Part print with two shaded views. Sizes in mm from the minimum x, y, z corner. A direction names the side the tool comes from. Coordinates: 2 decimals unless noted, no trailing zeros. Loops run counter-clockwise (first coordinate to the right, second up) from the corner with the lowest first, then second, coordinate; pieces in that order, holes last. Notation, with made-up numbers: (88.25, 16) -> (125.25, 16) arc R13 cw to (125.25, 40) -> close; hole circle Ø4 at (89, 0.25). An arc over 180 degrees is marked (long way). Write each question's results on one line, items separated by ' | '.
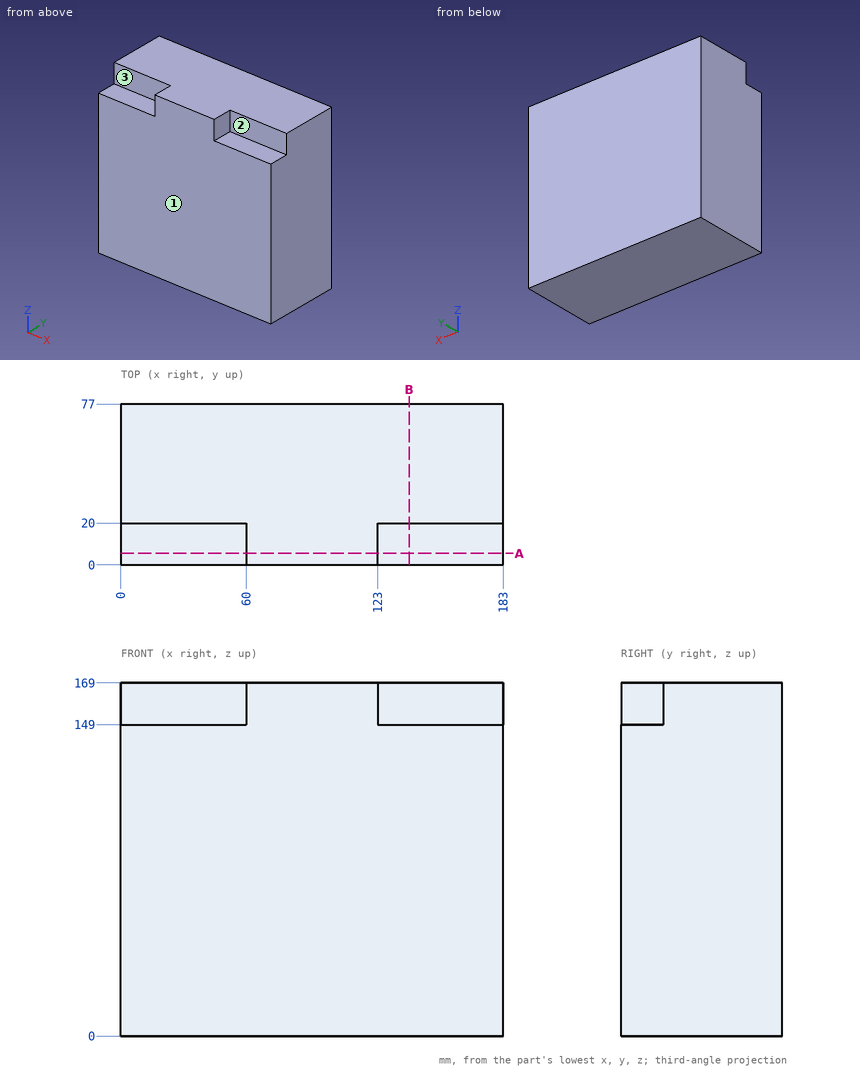
Q1. Which spindle directions (+Z, -Z, +X, -X, +Y, -Y) get a long thin tool onto all of the face, cutting with end or side? Do the marked faces 1, 2 and 3. Say none if no direction does.
Results are:
face 1: +Z, -Z, +X, -X, -Y | face 2: +Z, +X, -Y | face 3: +Z, -X, -Y
Q2. Drop flat-ended pins along their axis: pin 1 (6 mm diameter, centred on y = 12.5, z = 154.5, fed in from -X); pin 2 (22 mm diameter, centred on x = 24, y = 6.5, fed in from +Z); pin 3 (10 mm diameter, centred on y = 13.5, z = 162.5, fed in from +X). Give the stop position or say it passes through.
Results are:
pin 1: x = 60 | pin 2: z = 149 | pin 3: x = 123
Q3. Cut at A-A on y = 5.5. Write the cut outline in (x, z).
Results are:
outline: (0, 0) -> (183, 0) -> (183, 149) -> (123, 149) -> (123, 169) -> (60, 169) -> (60, 149) -> (0, 149) -> close
Q4. Wall check: L1, parallel to Z at x = 176.5, y = 6. Give the ranges that are in metal, low to high. Write a range as from..to.
Results are:
L1: 0..149
Q5. Cut at B-B on x = 138. Write the cut outline in (y, z).
Results are:
outline: (0, 0) -> (77, 0) -> (77, 169) -> (20, 169) -> (20, 149) -> (0, 149) -> close
